Verification items for the finished model (mm, model axes). Face numbers are marked on the shaded views. A direction names the side the tool comes from. Coordinates: 2 decimals unless noted, no trailing zeros. Loops run counter-clockwise (first coordinate to the right, second up) from the corner with the lowest first, then second, coordinate; pieces in that order, holes last. Notation, with made-up numbers: (3.5, 76.5) - (22.5, 76.5) arc R34 cw to (22.5, 114.5) - close; hole circle Ø7 at (45, 58.5). An arc over 180 degrees is marked (long way). One line per item, written item: value. Start each with the question number.
(1) Gauge pin test, flat ends, axial feed: P1, Ø10, axis at x = 8.5, y = 5, coming from the -Z side; P2, Ø3, axis at y = 19.5, z = 6, coming from the +X side; P3, Ø3, axis at x = -3.5, z = 7.5, coming from the -Y side; P4, Ø3, axis at x = 28, z = 7, coming from the -Y side. Record the tip position at first contact, or that the pin passes through.
(2) Set-up check for the marked faces 4, 5, 6 and 7: record each of +Z, -Z, +X, -X, +Y, -Y from which the full face is reachable in a straight line by a thin tool's end or side.
(3) Section check B-B (x = 16). Record the boundary of the cut face in (y, z), plus the area to 3 significant figures.
(4) Section check A-A (y = 19.36). Record the boundary of the cut face in (x, z).
(5) Section check C-C (z = 4). Count the separate pieces of the cut face and the enclosed holes in it, plus the area to 3 significant figures.
(6) Thickness scan on probe 1 along Y at (x, z) = (-6.5, 5); probe 2 along Y at (x, z) = (19.5, 1.25); probe 3 along X at (y, z) = (32, 8.5). Record the ranges inside material, lowest first. Write a range as [from, to].
(7) Draft check along Y on the marked faces 1, 2 and 3. Enter one of: +Y half, -Y half, draft (parallel to the pull), parting line (faces both ways), or undercut.
Autodesk Inventor part; units mm, degrees
ref_plane "YZ Plane" through (0, 0, 0) normal (1, 0, 0) x (0, 1, 0)
ref_plane "XZ Plane" through (0, 0, 0) normal (0, 1, 0) x (-1, 0, 0)
ref_plane "XY Plane" through (0, 0, 0) normal (0, 0, 1) x (1, 0, 0)
ref_plane "Arbeitsebene1" through (0, 0, 0) normal (0, 0, 1) x (1, 0, 0)
sketch "Skizze1" plane through (0, 0, 0) normal (0, 0, 1) x (1, 0, 0)
  arc A0 (12.7966, 13.5152) -> (12.2972, 14.0928) centre (11.6862, 13.06) ccw construction
  arc A1 (12.1755, 14.2862) -> (12.2972, 14.0928) centre (12.4245, 14.308) ccw construction
  line L0 (12.1755, 14.2862) -> (12.1453, 14.6318) construction
  arc A2 (12.1453, 14.6318) -> (11.8962, 14.86) centre (11.8962, 14.61) ccw construction
  line L1 (11.8962, 14.86) -> (11.4438, 14.86) construction
  arc A3 (11.4438, 14.86) -> (11.1947, 14.6318) centre (11.4438, 14.61) ccw construction
  line L2 (11.1947, 14.6318) -> (11.1627, 14.2652) construction
  arc A4 (11.0468, 14.0755) -> (11.1627, 14.2652) centre (10.9136, 14.287) ccw construction
  arc A5 (11.0468, 14.0755) -> (10.5759, 13.5152) centre (11.6862, 13.06) ccw construction
  arc A6 (10.3446, 13.36) -> (10.5759, 13.5152) centre (10.3446, 13.61) ccw construction
  line L3 (10.3446, 13.36) -> (9.67, 13.36) construction
  line L4 (9.67, 13.36) -> (9.17, 13.86) construction
  line L5 (9.17, 13.86) -> (9.17, 24.86) construction
  line L6 (9.17, 24.86) -> (9.67, 25.36) construction
  line L7 (9.67, 25.36) -> (10.3446, 25.36) construction
  arc A7 (10.5759, 25.2048) -> (10.3446, 25.36) centre (10.3446, 25.11) ccw construction
  arc A8 (10.5759, 25.2048) -> (11.0468, 24.6445) centre (11.6862, 25.66) ccw construction
  arc A9 (11.1627, 24.4548) -> (11.0468, 24.6445) centre (10.9136, 24.433) ccw construction
  line L8 (11.1627, 24.4548) -> (11.1947, 24.0882) construction
  arc A10 (11.1947, 24.0882) -> (11.4438, 23.86) centre (11.4438, 24.11) ccw construction
  line L9 (11.4438, 23.86) -> (11.8962, 23.86) construction
  arc A11 (11.8962, 23.86) -> (12.1453, 24.0882) centre (11.8962, 24.11) ccw construction
  line L10 (12.1453, 24.0882) -> (12.1755, 24.4338) construction
  arc A12 (12.2972, 24.6272) -> (12.1755, 24.4338) centre (12.4245, 24.412) ccw construction
  arc A13 (12.2972, 24.6272) -> (12.7966, 25.2048) centre (11.6862, 25.66) ccw construction
  arc A14 (13.0279, 25.36) -> (12.7966, 25.2048) centre (13.0279, 25.11) ccw construction
  line L11 (13.0279, 25.36) -> (14.17, 25.36) construction
  line L12 (14.17, 25.36) -> (14.17, 32.26) construction
  line L13 (14.17, 32.26) -> (13.57, 32.86) construction
  line L14 (13.57, 32.86) -> (10.17, 32.86) construction
  arc A15 (9.37, 32.86) -> (10.17, 32.86) centre (9.77, 33.16) ccw construction
  line L15 (9.37, 32.86) -> (4.77, 32.86) construction
  line L16 (4.77, 32.86) -> (4.17, 32.26) construction
  line L17 (4.17, 32.26) -> (4.17, 25.76) construction
  line L18 (4.17, 25.76) -> (4.57, 25.36) construction
  line L19 (4.57, 25.36) -> (4.57, 13.36) construction
  line L20 (4.57, 13.36) -> (4.17, 12.96) construction
  line L21 (4.17, 12.96) -> (4.17, 6.46) construction
  line L22 (4.17, 6.46) -> (4.77, 5.86) construction
  line L23 (4.77, 5.86) -> (13.57, 5.86) construction
  line L24 (13.57, 5.86) -> (14.17, 6.46) construction
  line L25 (14.17, 6.46) -> (14.17, 13.36) construction
  line L26 (14.17, 13.36) -> (13.0279, 13.36) construction
  arc A16 (12.7966, 13.5152) -> (13.0279, 13.36) centre (13.0279, 13.61) ccw construction
  line L27 (13.6528, 5.66) -> (4.6872, 5.66) construction
  line L28 (4.6872, 5.66) -> (3.97, 6.3772) construction
  line L29 (3.97, 6.3772) -> (3.97, 13.0428) construction
  line L30 (3.97, 13.0428) -> (4.37, 13.4428) construction
  line L31 (4.37, 13.4428) -> (4.37, 25.2772) construction
  line L32 (4.37, 25.2772) -> (3.97, 25.6772) construction
  line L33 (3.97, 25.6772) -> (3.97, 32.3428) construction
  line L34 (3.97, 32.3428) -> (4.6872, 33.06) construction
  line L35 (4.6872, 33.06) -> (9.4872, 33.06) construction
  arc A17 (9.4872, 33.06) -> (10.0528, 33.06) centre (9.77, 33.16) ccw construction
  line L36 (10.0528, 33.06) -> (13.6528, 33.06) construction
  line L37 (13.6528, 33.06) -> (14.37, 32.3428) construction
  line L38 (14.37, 32.3428) -> (14.37, 25.16) construction
  line L39 (14.37, 25.16) -> (13.0279, 25.16) construction
  arc A18 (13.0279, 25.16) -> (12.9816, 25.129) centre (13.0279, 25.11) ccw construction
  arc A19 (12.3991, 24.4551) -> (12.9816, 25.129) centre (11.6862, 25.66) ccw construction
  arc A20 (12.3991, 24.4551) -> (12.3747, 24.4164) centre (12.4245, 24.412) ccw construction
  line L40 (12.3747, 24.4164) -> (12.3445, 24.0708) construction
  arc A21 (11.8962, 23.66) -> (12.3445, 24.0708) centre (11.8962, 24.11) ccw construction
  line L41 (11.8962, 23.66) -> (11.4438, 23.66) construction
  arc A22 (10.9955, 24.0708) -> (11.4438, 23.66) centre (11.4438, 24.11) ccw construction
  line L42 (10.9955, 24.0708) -> (10.9634, 24.4373) construction
  arc A23 (10.9634, 24.4373) -> (10.9403, 24.4753) centre (10.9136, 24.433) ccw construction
  arc A24 (10.3909, 25.129) -> (10.9403, 24.4753) centre (11.6862, 25.66) ccw construction
  arc A25 (10.3909, 25.129) -> (10.3446, 25.16) centre (10.3446, 25.11) ccw construction
  line L43 (10.3446, 25.16) -> (9.7528, 25.16) construction
  line L44 (9.7528, 25.16) -> (9.37, 24.7772) construction
  line L45 (9.37, 24.7772) -> (9.37, 13.9428) construction
  line L46 (9.37, 13.9428) -> (9.7528, 13.56) construction
  line L47 (9.7528, 13.56) -> (10.3446, 13.56) construction
  arc A26 (10.3446, 13.56) -> (10.3909, 13.591) centre (10.3446, 13.61) ccw construction
  arc A27 (10.9403, 14.2447) -> (10.3909, 13.591) centre (11.6862, 13.06) ccw construction
  arc A28 (10.9403, 14.2447) -> (10.9634, 14.2827) centre (10.9136, 14.287) ccw construction
  line L48 (10.9634, 14.2827) -> (10.9955, 14.6492) construction
  arc A29 (11.4438, 15.06) -> (10.9955, 14.6492) centre (11.4438, 14.61) ccw construction
  line L49 (11.4438, 15.06) -> (11.8962, 15.06) construction
  arc A30 (12.3445, 14.6492) -> (11.8962, 15.06) centre (11.8962, 14.61) ccw construction
  line L50 (12.3445, 14.6492) -> (12.3747, 14.3036) construction
  arc A31 (12.3747, 14.3036) -> (12.3991, 14.2649) centre (12.4245, 14.308) ccw construction
  arc A32 (12.9816, 13.591) -> (12.3991, 14.2649) centre (11.6862, 13.06) ccw construction
  arc A33 (12.9816, 13.591) -> (13.0279, 13.56) centre (13.0279, 13.61) ccw construction
  line L51 (13.0279, 13.56) -> (14.37, 13.56) construction
  line L52 (14.37, 13.56) -> (14.37, 6.3772) construction
  line L53 (14.37, 6.3772) -> (13.6528, 5.66) construction
  line L54 (16.97, 24.8315) -> (24.85, 24.8315) construction
  line L55 (24.85, 36.23) -> (20.77, 36.23) construction
  line L56 (20.77, 36.23) -> (16.87, 36.23) construction
  line L57 (14.37, 25.66) -> (36.4731, 25.66)
  line L58 (14.37, 25.66) -> (36.4731, 25.66) construction
  line L59 (36.4731, 25.66) -> (36.4731, 33.86)
  line L60 (36.4731, 33.86) -> (18.5197, 33.86)
  line L61 (18.5197, 33.86) -> (14.3197, 38.06)
  line L62 (14.3197, 38.06) -> (3.97, 38.06)
  line L63 (-9.03, 33.06) -> (-9.03, 19.36)
  line L64 (-9.03, 19.36) -> (4.37, 19.36)
  line L65 (4.37, 19.36) -> (4.37, 25.2772)
  line L66 (4.37, 25.2772) -> (3.97, 25.6772)
  line L67 (3.97, 25.6772) -> (3.97, 33.06)
  line L68 (3.97, 33.06) -> (14.37, 33.06)
  line L69 (14.37, 33.06) -> (14.37, 25.66)
  circle A34 centre (-3.43, 19.36) radius 1.75 construction
  circle A35 centre (-0.2031, 19.36) radius 1.4
  circle A36 centre (60.62, 30.4425) radius 2.45
  circle A37 centre (35.7803, 19.36) radius 2.45
  circle A38 centre (60.62, 8.3286) radius 2.45
  line L70 (29.0574, 13.415) -> (26.7455, 13.415)
  line L71 (26.7455, 13.415) -> (26.7455, 10.1303)
  arc A39 (26.7455, 9.327) -> (26.7455, 10.1303) centre (28.0867, 9.7286) ccw
  line L72 (26.7455, 9.327) -> (26.7455, 5.8628)
  line L73 (26.7455, 5.8628) -> (35.12, 4.36)
  line L74 (35.12, 4.36) -> (65.12, 4.36)
  line L75 (65.12, 4.36) -> (65.12, 34.36)
  line L76 (65.12, 34.36) -> (35.12, 34.36)
  line L77 (35.12, 34.36) -> (26.7455, 32.9029)
  line L78 (26.7455, 32.9029) -> (26.7455, 29.4442)
  arc A40 (26.7455, 28.6409) -> (26.7455, 29.4442) centre (28.0867, 29.0425) ccw
  line L79 (26.7455, 28.6409) -> (26.7455, 25.3561)
  line L80 (26.7455, 25.3561) -> (29.0574, 25.3561)
  line L81 (29.0574, 25.3561) -> (29.0574, 13.415)
  circle A41 centre (50.12, 19.36) radius 10.5
  circle A42 centre (33.0867, 29.0425) radius 1.4
  circle A43 centre (33.0867, 9.7286) radius 1.4
  line L82 (36.7731, 34.36) -> (36.7731, 25.3561)
  line L83 (36.7731, 13.415) -> (36.7731, 4.36)
  circle A44 centre (33.0867, 29.0425) radius 1.4
  circle A45 centre (28.0867, 29.0425) radius 1.4
  line L84 (3.97, 38.06) -> (-1.03, 33.06)
  line L85 (3.97, 38.06) -> (11.0411, 38.06) construction
  line L86 (-1.03, 33.06) -> (-9.03, 33.06)
  point P0 (0, 0)
  point P1 (1.1969, 19.36)
  point P2 (-1.6031, 19.36)
  dimension "d0" = 0.2
  dimension "d2" = 5
  dimension "d4" = 13
  dimension "d5" = 2.8
  dimension "d7" = 0.5
  dimension "d8" = 3.5
  dimension "d19" = 0.3
  dimension "d20" = 0.5
  dimension "d21" = 135
  dimension "d28" = 8.8269
extrude "Extrusion1" add sketch "Skizze1" along normal blind 10 contours L69 L68 L67 L66 L65 L64 A35 L63 L86 L84 L62 L61 L60 L77 L78 A45 L79 L57 | L79 A40 L78 L77 L60 L59 L57
sketch "Skizze2" plane through (-9.03, 19.36, 0) normal (-1, 0, 0) x (0, 0, 1)
  circle A0 centre (12.1869, 10) radius 1.75
  line L0 (0, 13.7) -> (0, 0)
  line L1 (0, 0) -> (10, 0)
  line L2 (10, 13.7) -> (10, 0)
  line L3 (0, 13.7) -> (10, 13.7)
  circle A1 centre (5, 10) radius 1.5
  point P0 (0, -19.36)
  dimension "d11" = 3
hole "Bohrung1" at (-9.03, 29.36, 5) direction (1, 0, 0) diameter 3 depth 20 tip angle 118 counterbore diameter 6 counterbore depth 4
sketch "Skizze3" plane through (-9.03, 33.06, 0) normal (0, 1, 0) x (1, 0, 0)
  line L0 (4.1, -9.9) -> (4.1, 19.6933)
  line L1 (7.1, -9.9) -> (7.1, 19.6933)
  circle A0 centre (5.5663, -8.2216) radius 1.4
  point P0 (9.03, 0)
  dimension "d22" = 2.8
extrude "Extrusion2" cut sketch "Skizze3" against normal blind 10
mirror "Spiegeln2" about plane through (-9.03, 19.36, 0) normal (0, -1, 0) of "Extrusion1", "Bohrung1", "Extrusion2"
sketch "Skizze4" plane through (0, 0, 0) normal (0, 0, -1) x (-1, 0, 0)
  circle A0 centre (0.2031, 19.36) radius 1.4
  circle A1 centre (-28.0867, 9.6775) radius 1.4
  circle A2 centre (-33.0867, 9.6775) radius 1.4
  line L0 (-4.37, 13.4428) -> (-4.37, 25.2772)
  line L1 (-4.37, 13.4428) -> (-3.97, 13.0428)
  line L2 (-3.97, 13.0428) -> (-3.97, 5.66)
  line L3 (-3.97, 5.66) -> (-14.37, 5.66)
  line L4 (-14.37, 5.66) -> (-14.37, 13.06)
  line L5 (-14.37, 13.06) -> (-36.4731, 13.06)
  line L6 (-36.4731, 13.06) -> (-36.4731, 4.86)
  line L7 (-36.4731, 4.86) -> (-18.5197, 4.86)
  line L8 (-18.5197, 4.86) -> (-14.3197, 0.66)
  line L9 (-14.3197, 0.66) -> (-3.97, 0.66)
  line L10 (-3.97, 0.66) -> (1.03, 5.66)
  line L11 (1.03, 5.66) -> (9.03, 5.66)
  line L12 (9.03, 33.06) -> (9.03, 5.66)
  line L13 (1.03, 33.06) -> (9.03, 33.06)
  line L14 (-3.97, 38.06) -> (1.03, 33.06)
  line L15 (-14.3197, 38.06) -> (-3.97, 38.06)
  line L16 (-18.5197, 33.86) -> (-14.3197, 38.06)
  line L17 (-36.4731, 33.86) -> (-18.5197, 33.86)
  line L18 (-36.4731, 25.66) -> (-36.4731, 33.86)
  line L19 (-14.37, 25.66) -> (-36.4731, 25.66)
  line L20 (-14.37, 33.06) -> (-14.37, 25.66)
  line L21 (-3.97, 33.06) -> (-14.37, 33.06)
  line L22 (-3.97, 25.6772) -> (-3.97, 33.06)
  line L23 (-4.37, 25.2772) -> (-3.97, 25.6772)
  circle A3 centre (-33.0867, 29.0425) radius 1.4
  circle A4 centre (-28.0867, 29.0425) radius 1.4
  line L24 (-3.2969, 21.3807) -> (0.2031, 23.4015)
  line L25 (0.2031, 23.4015) -> (3.7031, 21.3807)
  line L26 (3.7031, 21.3807) -> (3.7031, 17.3393)
  line L27 (3.7031, 17.3393) -> (0.2031, 15.3185)
  line L28 (0.2031, 15.3185) -> (-3.2969, 17.3393)
  line L29 (-3.2969, 17.3393) -> (-3.2969, 21.3807)
  point P0 (0, 0)
  dimension "d25" = 7
extrude "Extrusion3" cut sketch "Skizze4" against normal blind 5 contours A0 | L24 L25 L26 L27 L28 L29
properties part number "30_Cube_Cube_Z_Focus_MGN_NEMA_belt_pushing_slide_v3"
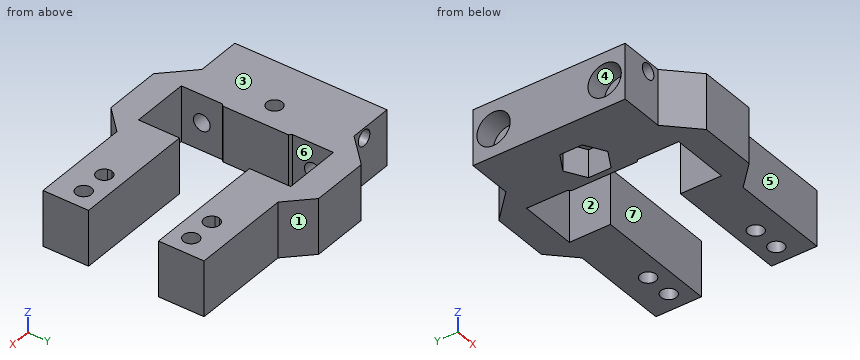
Responses:
1. P1: stops at z = 0
1. P2: stops at x = 4.37
1. P3: stops at y = 5.66
1. P4: stops at y = 4.86
2. face 4: -X
2. face 5: +Z, -Z, +X, -Y
2. face 6: +Z, -Z
2. face 7: +Z, -Z, +X
3. outline: (2.34, 0) - (13.06, 0) - (13.06, 10) - (2.34, 10) - close; (25.66, 0) - (36.38, 0) - (36.38, 10) - (25.66, 10) - close
3. area: 214 mm²
4. outline: (-9.03, 0) - (-3.7, 0) - (-3.7, 5) - (-1.6, 5) - (-1.6, 10) - (-9.03, 10) - close; (1.2, 5) - (3.3, 5) - (3.3, 0) - (4.37, 0) - (4.37, 10) - (1.2, 10) - close
5. separate pieces: 3
5. enclosed holes: 5
5. area: 717 mm²
6. probe 1: y = [5.66, 6.36], [12.36, 26.36], [32.36, 33.06]
6. probe 2: y = [4.86, 13.06], [25.66, 33.86]
6. probe 3: x = [-9.03, -4.84], [-2.09, 3.97], [14.37, 36.47]
7. face 1: +Y half
7. face 2: undercut
7. face 3: draft
